from build123d import *

# Parameters (mm, degrees)
SKETCH1_R               = 10.65
BOSS_EXTRUDE1_DEPTH     = 24
BOSS_EXTRUDE2_DEPTH     = 4
CUT_EXTRUDE1_DEPTH      = 52.962056715
CUT_EXTRUDE1_DEPTH_BACK = 52.962056715
SKETCH3_R               = 7
FILLET1_R               = 6


with BuildPart() as part:
    # Sketch1 → Boss-Extrude1 (new, symmetric)
    with BuildSketch(Plane(origin=(0, 0, 0), x_dir=(1, 0, 0), z_dir=(0, 1, 0))):
        with Locations(Location((0, 0, 0), (0, 0, 270))):
            Circle(SKETCH1_R)
    extrude(amount=BOSS_EXTRUDE1_DEPTH, both=True)

    # Sketch2 → Boss-Extrude2 (add, symmetric)
    with BuildSketch(Plane(origin=(0, 0, 0), x_dir=(1, 0, 0), z_dir=(0, 1, 0))):
        Polygon((13.066755915, 7.388722704), (0.134556394, 15.010503919), (-12.932199521, 7.621781215), (-13.066755915, -7.388722704), (-0.134556394, -15.010503919), (12.932199521, -7.621781215), align=None)
    extrude(amount=BOSS_EXTRUDE2_DEPTH, both=True)

    # Sketch3 → Cut-Extrude1 (cut, two sides: drawn at the far end of the back side and taken through both)
    with BuildSketch(Plane(origin=(0, 24, 0), x_dir=(1, 0, 0), z_dir=(0, 1, 0)).offset(-CUT_EXTRUDE1_DEPTH_BACK)):
        with Locations(Location((0, 0, 0), (0, 0, 270))):
            Circle(SKETCH3_R)
    extrude(amount=CUT_EXTRUDE1_DEPTH + CUT_EXTRUDE1_DEPTH_BACK, mode=Mode.SUBTRACT)

    # Fillet1
    # the kernel refuses this fillet: 6 mm, written as the material it takes off along each edge
    with BuildSketch(Plane(origin=(0, -24, 0), x_dir=(0, 0, 1), z_dir=(-1, 0, 0))) as fillet1_piece_1:
        with BuildLine():
            CenterArc((13, 5.520643078), FILLET1_R, 180, 66.941755912)
            Line((7, 5.520643078), (6.88, 5.520643078))
            Line((6.88, 5.520643078), (6.88, 0))
            Line((6.88, 0), (7, -0.12))
            ThreePointArc((7, -0.12), (8.825, -0.12), (10.603, -0.110412862))
            Line((10.603, -0.110412862), (10.65, 0))
        make_face()
    revolve(axis=Axis((0, -24, 0), (0, 1, 0)), mode=Mode.SUBTRACT)


solid = part.part
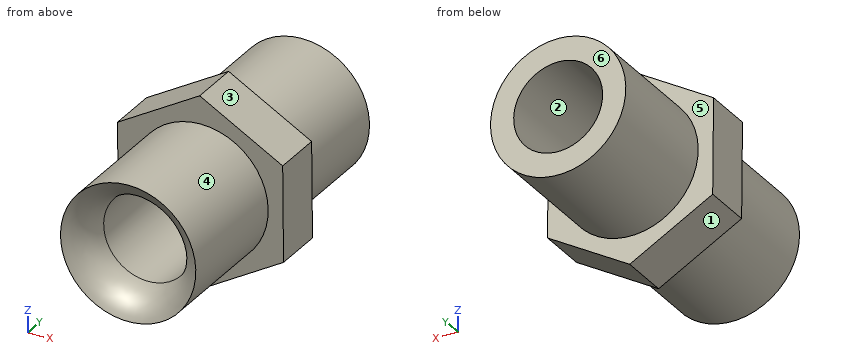
The model under review builds one solid part; all positions refer to its coordinate system, in mm. Face numbers are marked on the shaded views. A direction names the side the tool comes from. Give positions to 0.01 mm unless a question says otherwise; leave off trailing zeros. Loops run counter-clockwise (first coordinate to the right, second up) from the corner with the lowest first, then second, coordinate; pieces in that order, holes last. Notation, with made-up numbers: (-17, 59) -> (3, 59) arc R16 cw to (3, 74) -> close; hole circle Ø2 at (10, 32.5). An arc over 180 degrees is marked (long way). Write each question's results on one line, items separated by ' | '.
1) Take a section at A-A, the plane y = 3.5. Give the boundary of the cut face in (x, z), plus the area to 3 significant figures.
Conclusion:
outline: (-13.07, 7.39) -> (-12.93, -7.62) -> (0.13, -15.01) -> (13.07, -7.39) -> (12.93, 7.62) -> (-0.13, 15.01) -> close; hole circle Ø14 at (0, 0) | area: 431 mm^2
2) Take a section at B-B, the plane z = 0. Give the boundary of the cut face in (x, y).
Conclusion:
outline: (-13, -4) -> (-10.65, -4) -> (-10.65, -24) arc R6 ccw to (-7, -18.48) -> (-7, 24) -> (-10.65, 24) -> (-10.65, 4) -> (-13, 4) -> close; (7, -18.48) arc R6 ccw to (10.65, -24) -> (10.65, -4) -> (13, -4) -> (13, 4) -> (10.65, 4) -> (10.65, 24) -> (7, 24) -> close
3) Tool access review of the marked faces 4, 5 and 6: name each direction out of +Z, -Z, +X, -X, +Y, -Y from which nothing blocks a thin tool from reaching the whole face with its end or side.
Conclusion:
face 4: -Y | face 5: +Y | face 6: +Z, -Z, +X, -X, +Y
4) For line 1 along X through (y, z) = (-6.5, 0); line 2 along X through (y, z) = (-1, 4); line 3 along Y through (x, z) = (1.5, -11), list the stretches that pass through material, from the lowest coordinate up. Write a range as from..to.
Conclusion:
line 1: x = -10.65..-7, 7..10.65 | line 2: x = -13.04..-5.74, 5.74..12.96 | line 3: y = -4..4
5) Take a section at C-C, the plane x = -11.5. Give the boundary of the cut face in (y, z), plus the area to 3 significant figures.
Conclusion:
outline: (-4, -8.43) -> (4, -8.43) -> (4, 8.31) -> (-4, 8.31) -> close | area: 134 mm^2
6) Draft analysis for pull direction X (two halves, no side actions). For the marked faces 1, 2 and 3, state which applies: pulls with the +X half, pulls with the -X half, needs draft (parallel to the pull), parting line crosses it, or undercut.
Conclusion:
face 1: pulls with the -X half | face 2: undercut | face 3: pulls with the +X half
7) Insertion check: pin 1 Ø8 at (x, y) = (5.5, -5) entering from +Z; pin 2 Ø3 at (x, y) = (7, -11) entering from -Z; pin 3 Ø3 at (y, z) = (-9.5, 10.5) entering from +X. Each pin has a flat end and moves straight along its axis. Give the tip position at first contact, or say it passes through.
Conclusion:
pin 1: stops at z = 14.01 | pin 2: stops at z = -9.12 | pin 3: stops at x = 5.69
